The figure shows three views and two pictorial views of one solid part (mm, origin at its lowest corner). Answer the questions. Give positions to 0.01 mm unless a question says otherwise; leave off trailing zeros. Loops run counter-clockwise (first coordinate to the right, second up) from the corner with the lowest first, then second, coordinate; pieces in that order, holes last. Notation, with made-up numbers: (-11, 33) - (34, 33) arc R8 ccw to (34, 44) - close; hole circle Ø7 at (-38.5, 47). An arc over 180 degrees is marked (long way). One line per question, with ' | ' between items.
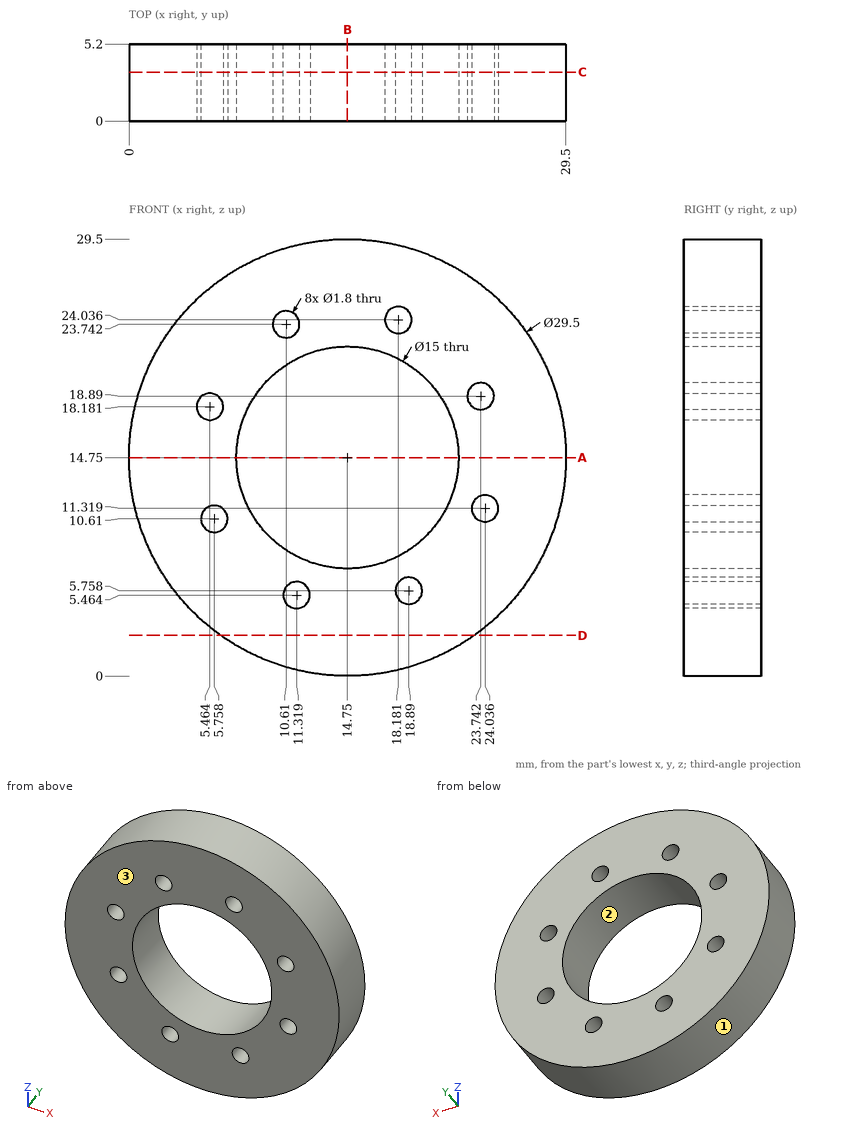
1. Find section C-C on y = 3.3. State how many separate pieces and enclosed holes the cut face has.
Evaluation:
separate pieces: 1 | enclosed holes: 9
2. Flat-ended cylindrical pins translate along their axes: pin 1 (1 mm diameter, centred on y = 4.5, z = 13.5, fed in from -X); pin 2 (1 mm diameter, centred on x = 26, y = 3, fed in from -Z). Find the tip coordinate at first contact, or state that the pin passes through.
Evaluation:
pin 1: x = 0.02 | pin 2: z = 4.65
3. Find section D-D on z = 2.75. Write down the section's boundary in (x, y).
Evaluation:
outline: (6.17, 0) - (23.33, 0) - (23.33, 5.2) - (6.17, 5.2) - close
4. Determine the mould class of the marked faces 1, 2 and 3 for opening direction Z: +Z half, -Z half, draft (parallel to the pull), parting line (faces both ways), or undercut.
Evaluation:
face 1: parting line | face 2: undercut | face 3: draft
5. Find section B-B on x = 14.75. Write down the section's boundary in (y, z), then the cut area to 3 significant figures.
Evaluation:
outline: (0, 0) - (5.2, 0) - (5.2, 7.25) - (0, 7.25) - close; (0, 22.25) - (5.2, 22.25) - (5.2, 29.5) - (0, 29.5) - close | area: 75.4 mm2
6. Consider L1, parallel to X at y = 1.05, z = 6 (1 decimal); L2, parallel to X at y = 1.5, z = 18.75 (1 decimal); L3, parallel to Z at x = 18.75, y = 4.05 (1 decimal). Determine where each line is inside the solid, lowest interval first.
Evaluation:
L1: 2.9 to 10.6, 12 to 18, 19.8 to 26.6 | L2: 0.6 to 4.8, 6.2 to 8.4, 21.1 to 22.9, 24.6 to 28.9 | L3: 0.6 to 4.9, 6.6 to 8.4, 21.1 to 23.3, 24.7 to 28.9
7. Find section A-A on z = 14.75. Write down the section's boundary in (x, y), then the cut area to 3 significant figures.
Evaluation:
outline: (0, 0) - (7.25, 0) - (7.25, 5.2) - (0, 5.2) - close; (22.25, 0) - (29.5, 0) - (29.5, 5.2) - (22.25, 5.2) - close | area: 75.4 mm2
